Build history of the part. All positions in model axes, mm. A direction names the side the tool comes from. Give positions to 0.01 mm unless a question says otherwise; leave off trailing zeros. Loops run counter-clockwise (first coordinate to the right, second up) from the corner with the lowest first, then second, coordinate; pieces in that order, holes last. Notation, with made-up numbers: (-2.5, 83) - (2.5, 83) arc R22 ccw to (2.5, 117) - close; hole circle Ø1 at (16, 16). An arc over 180 degrees is marked (long way). Return JSON: item names as keys, results as strings. Group by question number.
1) Mould opens along X. For faces 1 (the face through (-27.5, -22, 4)), 2 (the face through (17.5, -10, 2)), 3 (the face through (-19.75, -20, 4)) say: released by +X, released by -X, zero draft, split by the parting line, or undercut.
2) Drill centre lines: probe 1 along X at (y, z) = (-19.5, 5.5); probe 2 along Y at (x, z) = (22, 6.5); probe 3 along Y at (x, z) = (19, 6.75). Where is each one in solid material? Low to high. Write a range as from..to.
3) Slice it at D-D (y = 14). List the corners of the cut face in (x, z).
4) Slice it at C-C (y = -23.5). List the corners of the cut face in (x, z), and give its area (3 significant figures).
5) 3-axis set-ups, long thin cutter, end or side, ignore diameter. For faces 4 (the face through (-1.756, -7.907, 1.972)), 5 (the face through (-18, -25, 4)), 6 (the face through (23.894, -20.479, 6.37)): which of +Z, -Z, +X, -X, +Y, -Y reach the whole face in a straight line?
6) Drop flat-ended pins along their axis: pin 1 (1.8 mm diameter, centred on y = -27.5, z = 4.5, fed in from +X); pin 2 (3 mm diameter, centred on y = -6.5, z = 3, fed in from +X); pin 3 (4.5 mm diameter, centred on x = 22, z = 3.5, fed in from +Y); pin 4 (2.5 mm diameter, centred on x = -10.25, y = 5.92, fed in from -Z). Give the stop position or say it passes through.
7) Slice it at B-B (x = -9.5). List the corners of the cut face in (y, z).
8) Slice it at A-A (x = 0). List the corners of the cut face in (y, z).
```python
from build123d import *

# Parameters (mm, degrees)
ESQUISSE1_R             = 8.1
ESQUISSE1_R_2           = 1.65
BOSS_EXTRU_1_DEPTH      = 4
BOSS_EXTRU_2_DEPTH      = 4
CHANFREIN1_SIZE         = 2.5
ENL_V_MAT_EXTRU_1_DEPTH = 3
ESQUISSE5_R             = 1.6
ENL_V_MAT_EXTRU_2_DEPTH = 47.395042839


with BuildPart() as part:
    # Esquisse1 → Boss.-Extru.1 (new body)
    with BuildSketch(Plane.XY):
        with BuildLine():
            Line((-27.5, -19), (-27.5, -25))
            Line((-27.5, -25), (-7.5, -25))
            Line((-7.5, -25), (-7.5, -31))
            Line((-7.5, -31), (7.5, -31))
            Line((7.5, -31), (7.5, -25))
            Line((7.5, -25), (27.5, -25))
            Line((27.5, -25), (27.5, -19))
            Line((27.5, -19), (17.5, -19))
            Line((17.5, -19), (17.5, 0))
            ThreePointArc((17.5, 0), (0, 17.5), (-17.5, 0))
            Line((-17.5, 0), (-17.5, -19))
            Line((-17.5, -19), (-27.5, -19))
        make_face()
        Circle(ESQUISSE1_R, mode=Mode.SUBTRACT)
        with Locations((-10.25, 5.917840259)):
            Circle(ESQUISSE1_R_2, mode=Mode.SUBTRACT)
        with Locations((10.25, 5.917840259)):
            Circle(ESQUISSE1_R_2, mode=Mode.SUBTRACT)
        with Locations((0, -11.835680518)):
            Circle(ESQUISSE1_R_2, mode=Mode.SUBTRACT)
    extrude(amount=BOSS_EXTRU_1_DEPTH)

    # Esquisse2 → Boss.-Extru.2 (add)
    with BuildSketch(Plane.XY.offset(4)):
        Polygon((-27.5, -25), (-7.5, -25), (-7.5, -31), (7.5, -31), (7.5, -25), (27.5, -25), (27.5, -19), (-27.5, -19), align=None)
    extrude(amount=BOSS_EXTRU_2_DEPTH)

    # Chanfrein1
    chanfrein1_edges = [part.edges().sort_by_distance(p)[0] for p in [
        (0, -19, 4),
    ]]
    chamfer(chanfrein1_edges, length=CHANFREIN1_SIZE)

    # Esquisse3 → Enlèv. mat.-Extru.1 (cut)
    with BuildSketch(Plane(origin=(0, -19, 0), x_dir=(1, 0, 0), z_dir=(0, 1, 0))):
        Polygon((19.75, -2.41228676), (22.5, -0.824573519), (25.25, -2.41228676), (25.25, -5.58771324), (22.5, -7.175426481), (19.75, -5.58771324), align=None)
        Polygon((-22.5, -0.824573519), (-25.25, -2.41228676), (-25.25, -5.58771324), (-22.5, -7.175426481), (-19.75, -5.58771324), (-19.75, -2.41228676), align=None)
    extrude(amount=-ENL_V_MAT_EXTRU_1_DEPTH, mode=Mode.SUBTRACT)

    # Esquisse5 → Enlèv. mat.-Extru.2 (cut, through all)
    with BuildSketch(Plane(origin=(0, -19, 0), x_dir=(1, 0, 0), z_dir=(0, 1, 0))):
        with Locations(Location((-22.5, -4, 0), (0, 0, 270))):
            Circle(ESQUISSE5_R)
        with Locations(Location((22.5, -4, 0), (0, 0, 180))):
            Circle(ESQUISSE5_R)
    extrude(amount=-ENL_V_MAT_EXTRU_2_DEPTH, mode=Mode.SUBTRACT)


solid = part.part
```
Results:
{
 "1": {"face 1": "released by -X", "face 2": "released by +X", "face 3": "undercut"},
 "2": {"probe 1": "-27.5..-25.25, -19.75..19.75, 25.25..27.5", "probe 2": "-25..-22", "probe 3": "-25..-19"},
 "3": {"outline": "(-10.5, 0) - (10.5, 0) - (10.5, 4) - (-10.5, 4) - close"},
 "4": {"outline": "(-27.5, 0) - (27.5, 0) - (27.5, 8) - (-27.5, 8) - close; hole circle Ø3.2 at (-22.5, 4); hole circle Ø3.2 at (22.5, 4)", "area": "424 mm2"},
 "5": {"face 4": "+Z, -Z", "face 5": "+Z, -Z, -X, -Y", "face 6": "+Y"},
 "6": {"pin 1": "x = 7.5", "pin 2": "x = 17.5", "pin 3": "y = -19", "pin 4": "through"},
 "7": {"outline": "(-25, 0) - (4.45, 0) - (4.45, 4) - (-16.5, 4) - (-19, 6.5) - (-19, 8) - (-25, 8) - close; (7.39, 0) - (14.7, 0) - (14.7, 4) - (7.39, 4) - close"},
 "8": {"outline": "(-31, 0) - (-13.49, 0) - (-13.49, 4) - (-16.5, 4) - (-19, 6.5) - (-19, 8) - (-31, 8) - close; (-10.19, 0) - (-8.1, 0) - (-8.1, 4) - (-10.19, 4) - close; (8.1, 0) - (17.5, 0) - (17.5, 4) - (8.1, 4) - close"}
}
